Read the model definition and answer for the solid it produces. Units are mm, in the model's axes. A direction names the side the tool comes from. Round coordinates to 2 decimals unless told otherwise and drop trailing zeros. Order: outer loops, then holes, each group sorted by start corner. A loop starts at its lowest first (then second) coordinate and runs counter-clockwise, first axis right, second up. Notation, with made-up numbers: (40.5, 15.25) - (48.5, 15.25) arc R4 ccw to (48.5, 21.25) - close; hole circle Ø7 at (-7, 26.25). An arc over 180 degrees is marked (long way). One line per question, with ' | ' between items. Start each with the question number.
1) The part is cut by section B-B, the plane y = 0. Give the vertices of the cut face in (x, z), plus the area to 3 significant figures.
2) Flat-ended cylindrical pins translate along their axes: pin 1 (1 mm diameter, centred on y = -2, z = 10.5, fed in from +X); pin 2 (5 mm diameter, centred on y = -8, z = 12.5, fed in from -X); pin 3 (2.5 mm diameter, centred on x = 0.5, y = -9, fed in from -Z); pin 4 (4 mm diameter, centred on x = 0, y = 16, fed in from +Z). Find the tip coordinate at first contact, or state that the pin passes through.
3) The part is cut by section D-D, the plane z = 5.5. Give the vertices of the cut face in (x, y).
4) Straight lines are drawn through the part: line 1 (Y direction, x = 0, z = 6.5); line 2 (Y direction, x = 0, z = 13.5); line 3 (Y direction, x = -3, z = 11.5). For each, find the intervals that lie inside material, in ascending order. Write a range as from..to.
5) For faces 1 (the flat face through (3, 1, 8)), 2 (the flat face through (-2.25, 8, 13)), 3 (the flat face through (2.25, -8, 13)), 4 (the cylindrical face through (-0.46, 19.47, 7.4)), determine the directions among +Z, -Z, +X, -X, +Y, -Y from which every point of the face is accessible in a straight line to the end or side of a thin tool.
6) The part is cut by section A-A, the plane z = 10. Give the vertices of the cut face in (x, y), plus the area to 3 significant figures.
7) The part is cut by section C-C, the plane x = 0. Give the vertices of the cut face in (y, z).
8) The mould has two halves that part along Y. Classify faces 5 (the cylindrical face through (-0.37, 14.34, 7.4)), 6 (the flat face through (2, -15, 0)), 7 (the cylindrical face through (-4, 0, 11)): pulls with the +Y half, pulls with the -Y half, needs draft (parallel to the pull), parting line crosses it, or undercut.
from build123d import *

# Parameters (mm, degrees)
CYLINDER001_R     = 1.7
CYLINDER001_DEPTH = 15
CYLINDER_R        = 3.5
CYLINDER_DEPTH    = 15
CYLINDER002_R     = 2.9
CYLINDER002_DEPTH = 7
BOX_W             = 4.5
BOX_H             = 28
BOX_DEPTH         = 4.5
CYLINDER003_R     = 4
CYLINDER003_DEPTH = 7


with BuildPart() as leg_inner:
    # Cylinder001 → Cylinder001 (new body)
    with BuildSketch(Plane(origin=(0, -16, 0), x_dir=(1, 0, 0), z_dir=(0, 0, 1))):
        Circle(CYLINDER001_R)
    extrude(amount=CYLINDER001_DEPTH)


with BuildPart() as leg_outer:
    # Cylinder → Cylinder (new body)
    with BuildSketch(Plane(origin=(0, -16, 0), x_dir=(1, 0, 0), z_dir=(0, 0, 1))):
        Circle(CYLINDER_R)
    extrude(amount=CYLINDER_DEPTH)


with BuildPart() as rough_leg_r:
    # Cut001 base: copy of leg_outer
    add(leg_outer.part)

    # Cut001: cut leg_inner
    add(leg_inner.part, mode=Mode.SUBTRACT)


with BuildPart() as rough_leg_r_1:
    # Cut001 placement: moved
    add(rough_leg_r.part.moved(Location((0, 32, 0))))


with BuildPart() as tubing_bore:
    # Cylinder002 → Cylinder002 (new body)
    with BuildSketch(Plane.XY.offset(8)):
        Circle(CYLINDER002_R)
    extrude(amount=CYLINDER002_DEPTH)


with BuildPart() as rough_arch:
    # Box → Box (new body)
    with BuildSketch(Plane(origin=(-2.25, -14, 10.5), x_dir=(1, 0, 0), z_dir=(0, 0, 1))):
        with Locations((2.25, 14)):
            Rectangle(BOX_W, BOX_H)
    extrude(amount=BOX_DEPTH)


with BuildPart() as center:
    # Cylinder003 → Cylinder003 (new body)
    with BuildSketch(Plane.XY.offset(8)):
        Circle(CYLINDER003_R)
    extrude(amount=CYLINDER003_DEPTH)

    # Fusion: union rough_arch
    add(rough_arch.part)

    # Cut002: cut tubing_bore
    add(tubing_bore.part, mode=Mode.SUBTRACT)


with BuildPart() as rough_tubing_support:
    # Cut base: copy of leg_outer
    add(leg_outer.part)

    # Cut: cut leg_inner
    add(leg_inner.part, mode=Mode.SUBTRACT)

    # Fusion001: union rough_leg_r, center
    add(rough_leg_r_1.part)
    add(center.part)


solid = rough_tubing_support.part
Values:
1) outline: (-4, 8) - (-2.9, 8) - (-2.9, 15) - (-4, 15) - close; (2.9, 8) - (4, 8) - (4, 15) - (2.9, 15) - close | area: 15.4 mm^2
2) pin 1: stops at x = 3.71 | pin 2: stops at x = -2.25 | pin 3: stops at z = 10.5 | pin 4: stops at z = 15
3) outline: circle Ø7 at (0, -16); circle Ø7 at (0, 16); hole circle Ø3.4 at (0, -16); hole circle Ø3.4 at (0, 16)
4) line 1: y = -19.5..-17.7, -14.3..-12.5, 12.5..14.3, 17.7..19.5 | line 2: y = -19.5..-17.7, -14.3..-2.9, 2.9..14.3, 17.7..19.5 | line 3: y = -17.8..-14.2, -2.65..2.65, 14.2..17.8
5) face 1: -Z, +X, -X | face 2: +Z, -Z, -X | face 3: +Z, -Z, +X | face 4: -Z
6) outline: circle Ø8 at (0, 0); circle Ø7 at (0, -16); circle Ø7 at (0, 16); hole circle Ø5.8 at (0, 0); hole circle Ø3.4 at (0, -16); hole circle Ø3.4 at (0, 16) | area: 82.7 mm^2
7) outline: (-19.5, 0) - (-17.7, 0) - (-17.7, 15) - (-19.5, 15) - close; (-14.3, 0) - (-12.5, 0) - (-12.5, 10.5) - (-4, 10.5) - (-4, 8) - (-2.9, 8) - (-2.9, 15) - (-14.3, 15) - close; (2.9, 8) - (4, 8) - (4, 10.5) - (12.5, 10.5) - (12.5, 0) - (14.3, 0) - (14.3, 15) - (2.9, 15) - close; (17.7, 0) - (19.5, 0) - (19.5, 15) - (17.7, 15) - close
8) face 5: undercut | face 6: needs draft | face 7: undercut
